Geometry: final body of the model. Coordinates: model frame, mm. A direction names the side the tool comes from. Coordinates: 2 decimals unless noted, no trailing zeros. Loops run counter-clockwise (first coordinate to the right, second up) from the corner with the lowest first, then second, coordinate; pieces in that order, holes last. Notation, with made-up numbers: (-3, 15.5) -> (48, 15.5) arc R24 ccw to (48, 47.5) -> close; hole circle Ø5 at (19.25, -2.75). An arc over 180 degrees is marked (long way). One line per item, written item: value. Start each with the question number.
Item 1: Contact query for flat-ended pins moving along their axis: pin 1 Ø15 at (x, y) = (-19, 7) entering from -Z; pin 2 Ø12 at (y, z) = (-1.5, -20.5) entering from -X; pin 3 Ø10 at (y, z) = (-1, -10) entering from +X. Output: stop coordinate, or through.
Item 2: Section query A-A on y = 0. Return loops of the section in (x, z), then the cut area to 3 significant figures.
Item 3: Set-up query: faces 1 (the flat face through (-27, -4, -8)), 2 (the flat face through (-48, 12, -4)), 3 (the flat face through (-28, -3, -4)). Return all of +Z, -Z, +X, -X, +Y, -Y with unobstructed straight access to the full face (end or side cutting, diameter ignored); none if empty.
Item 4: Section query C-C on z = -4.5. Return loops of the section in (x, y), then the cut area to 3 significant figures.
Item 5: Ray query, probe 1 along Z at (x, y) = (-10, -9); probe 2 along X at (y, z) = (0.5, -15); probe 3 along X at (y, z) = (-2.5, -5). Return the intervals inside material, ascending. Write a range as from..to.
Item 6: Mould query, pull axis X, two halves, no side actions, for faces 4 (the cylindrical face through (7.79, 0.434, -15.593)), 5 (the flat face through (-7, 15, -6)), 6 (the cylindrical face through (27.19, 12.15, -38.53)). Classes: +X half, -X half, draft (parallel to the pull), parting line (faces both ways), or undercut.
Item 7: Section query D-D on y = 11. Return loops of the section in (x, z), then the cut area to 3 significant figures.
Item 8: Section query B-B on x = -25. Return loops of the section in (y, z).
from build123d import *

# Parameters (mm, degrees)
F1_DEPTH = 15
F3_DEPTH = 43.4455230334
F5_D     = 4
F6_R     = 10
F7_SIZE  = 5


with BuildPart() as f1:
    # F0 (on Front) → F1 (new body, symmetric)
    with BuildSketch(Plane.XZ):
        Polygon((0, 0), (-50, 0), (-50, -8), (-3.7304612652, -8), (26.0110249394, -43.4445230334), (32.1393804843, -38.3022221559), align=None)
    extrude(amount=F1_DEPTH, both=True)

    # F2 (on face) → F3 (cut, through all)
    with BuildSketch(Plane.XY):
        with BuildLine():
            ThreePointArc((-35, 3), (-38, 0), (-35, -3))
            Line((-35, -3), (-20, -3))
            ThreePointArc((-20, -3), (-17, 0), (-20, 3))
            Line((-20, 3), (-35, 3))
        make_face()
    extrude(amount=-F3_DEPTH, mode=Mode.SUBTRACT)

    # F5 (through all)
    with Locations(Plane(origin=(0, 0, 0), x_dir=(0, 1, 0), z_dir=(0.7660444431, 0, 0.6427876097))):
        with Locations((0, -15), (0, -35)):
            Hole(F5_D / 2)

    # F6
    f6_edges = [f1.edges().sort_by_distance(p)[0] for p in [
        (29.075203, 15, -40.873373),
        (29.075203, -15, -40.873373),
    ]]
    fillet(f6_edges, radius=F6_R)

    # F7
    f7_edges = [f1.edges().sort_by_distance(p)[0] for p in [
        (-50, -15, -4),
        (-50, 15, -4),
    ]]
    chamfer(f7_edges, length=F7_SIZE)


solid = f1.part
Reply:
1. pin 1: stops at z = -8
1. pin 2: stops at x = 1.72
1. pin 3: stops at x = 12.59
2. outline: (-50, -8) -> (-38, -8) -> (-38, 0) -> (-50, 0) -> close; (-17, -8) -> (-3.73, -8) -> (2.23, -15.1) -> (8.36, -9.96) -> (0, 0) -> (-17, 0) -> close; (4.8, -18.17) -> (15.08, -30.42) -> (21.21, -25.28) -> (10.93, -13.02) -> close; (17.65, -33.49) -> (26.01, -43.44) -> (32.14, -38.3) -> (23.78, -28.34) -> close
2. area: 538 mm²
3. face 1: -Z, -X, +Y, -Y
3. face 2: +Z, -Z, -X, +Y
3. face 3: +Z, -Z
4. outline: (-50, -10) -> (-45, -15) -> (3.78, -15) -> (3.78, 15) -> (-45, 15) -> (-50, 10) -> close; hole (-35, -3) -> (-20, -3) arc R3 ccw to (-20, 3) -> (-35, 3) arc R3 ccw to start
4. area: 1,470 mm²
5. probe 1: z = -8..0
5. probe 2: x = 2.14..2.45, 8.47..12.59
5. probe 3: x = -50..-36.66, -18.34..4.2
6. face 4: undercut
6. face 5: draft
6. face 6: +X half
7. outline: (-49, -8) -> (-3.73, -8) -> (24.73, -41.91) -> (30.85, -36.77) -> (0, 0) -> (-49, 0) -> close
7. area: 746 mm²
8. outline: (-15, -8) -> (-3, -8) -> (-3, 0) -> (-15, 0) -> close; (3, -8) -> (15, -8) -> (15, 0) -> (3, 0) -> close
